Source: CAD feature listing. Evaluate the final solid. Frame: model axes, mm. Round coordinates to 2 decimals unless told otherwise and drop trailing zeros. Write each loop counter-clockwise with the first axis right and the second up, starting at its lowest first coordinate (ties: lowest second). Pieces come first, ordered by that corner, then holes. Notation, with made-up numbers: M 76.25,67 L 130.25,67 A8 cw 130.25,74 Z; hole C 86.5,72 d4. An arc over 180 degrees is marked long. Answer in a Markdown table with one row per item. Add a question column.
Item 1: Contact query for flat-ended pins moving along their axis: pin 1 (1.5 mm diameter, centred on y = 2.5, z = -1, fed in from +X); pin 2 (1 mm diameter, centred on y = 3, z = 1, fed in from -X); pin 3 (1 mm diameter, centred on y = 2.5, z = 0.5, fed in from -X). Output: stop coordinate, or through.
Item 2: Cut plane A-A on z = 0.7. Return loops of the section in (x, y).
Item 3: Mould query, pull axis Y, two halves, no side actions, for faces 1 (the face through (0, 0, 1.3)), 2 (the face through (0, 0, -1.3)). Classes: released by +Y, released by -Y, zero draft, split by the parting line, or undercut.
Item 4: Material intervals for probe 1 along Y at (x, z) = (-1.25, 1.1); probe 2 along Z at (x, y) = (-0.8, 0); probe 3 along Z at (x, y) = (-0.8, 1.5), sorted ascending.
from build123d import *

# Parameters (mm, degrees)
SKETCH1_W                = 3.6
SKETCH1_H                = 4.4
EXTRUDE1_DEPTH           = 1.3
EXTRUDE1_TAPER           = 7
EXTRUDE1_OTHER_WAY_DEPTH = 1.3
EXTRUDE1_OTHER_WAY_TAPER = 7
FILLET1_R                = 0.2
SKETCH3_W                = 0.4
SKETCH3_H                = 0.2
SKETCH7_R                = 0.3
EXTRUDE2_DEPTH           = 0.1
SKETCH5_W                = 0.4
SKETCH5_H                = 0.2


with BuildPart() as part:
    # Sketch1 → Extrude1 (new body)
    with BuildSketch(Plane.XY):
        Rectangle(SKETCH1_W, SKETCH1_H)
    extrude(amount=EXTRUDE1_DEPTH, taper=EXTRUDE1_TAPER)

    # Sketch1 → Extrude1 other way (add)
    with BuildSketch(Plane.XY):
        Rectangle(SKETCH1_W, SKETCH1_H)
    extrude(amount=-EXTRUDE1_OTHER_WAY_DEPTH, taper=EXTRUDE1_OTHER_WAY_TAPER)

    # Fillet1
    fillet1_edges = [part.edges().sort_by_distance(p)[0] for p in [
        (-1.640380071, 0, -1.3),
        (0, -2.040380071, -1.3),
        (1.640380071, 0, 1.3),
        (0, 2.040380071, 1.3),
        (-1.640380071, 0, 1.3),
        (0, -2.040380071, 1.3),
        (1.640380071, 0, -1.3),
        (0, 2.040380071, -1.3),
    ]]
    fillet(fillet1_edges, radius=FILLET1_R)

    # Sweep4: sweep along a path in Sketch4
    with BuildLine(Plane(origin=(0, 0, 0), x_dir=(0, 0, -1), z_dir=(1, 0, 0))) as sweep4_path:
        Line((0, 2.061944248), (0, 2.307301205))
        ThreePointArc((0, 2.307301205), (-0.04178036, 2.429639038), (-0.149665454, 2.500863685))
        Line((-0.149665454, 2.500863685), (-1.150334546, 2.761080563))
        ThreePointArc((-1.150334546, 2.761080563), (-1.25821964, 2.83230521), (-1.3, 2.954643043))
        Line((-1.3, 2.954643043), (-1.3, 3.5))
    # Sketch3 → Sweep4 (sweep)
    with BuildSketch(Plane(origin=(0, 2.061944248, 0), x_dir=(-1, 0, 0), z_dir=(0, 1, 0))):
        with Locations((1.27, 0)):
            Rectangle(SKETCH3_W, SKETCH3_H)
        with Locations((-1.27, 0)):
            Rectangle(SKETCH3_W, SKETCH3_H)
    sweep(path=sweep4_path.line)

    # Sketch7 → Extrude2 (cut)
    with BuildSketch(Plane(origin=(0, 0, -1.3), x_dir=(-1, 0, 0), z_dir=(0, 0, -1))):
        with Locations((1.02, 1.4)):
            Circle(SKETCH7_R)
    extrude(amount=-EXTRUDE2_DEPTH, mode=Mode.SUBTRACT)

    # Sweep3: sweep along a path in Sketch8
    with BuildLine(Plane(origin=(0, 0, 0), x_dir=(0, 0, -1), z_dir=(1, 0, 0))) as sweep3_path:
        Line((-1.3, -3.5), (-1.3, -2.954643043))
        ThreePointArc((-1.3, -2.954643043), (-1.25821964, -2.83230521), (-1.150334546, -2.761080563))
        Line((-1.150334546, -2.761080563), (-0.149665454, -2.500863685))
        ThreePointArc((-0.149665454, -2.500863685), (-0.04178036, -2.429639038), (0, -2.307301205))
        Line((0, -2.307301205), (0, -2.061944248))
    # Sketch5 → Sweep3 (sweep)
    with BuildSketch(Plane(origin=(0, -2.061944248, 0), x_dir=(-1, 0, 0), z_dir=(0, 1, 0))):
        with Locations((1.27, 0)):
            Rectangle(SKETCH5_W, SKETCH5_H)
        Rectangle(SKETCH5_W, SKETCH5_H)
        with Locations((-1.27, 0)):
            Rectangle(SKETCH5_W, SKETCH5_H)
    sweep(path=sweep3_path.line)


solid = part.part
Results below:
| question | item | result |
|---|---|---|
| 1 | pin 1 | x = 1.76 |
| 1 | pin 2 | x = -1.47 |
| 1 | pin 3 | x = -1.79 |
| 2 | outline | M -1.71,-2.11 L 1.71,-2.11 L 1.71,2.11 L -1.71,2.11 Z; M -1.47,-2.75 L -1.07,-2.75 L -1.07,-2.54 L -1.47,-2.54 Z; M -1.47,2.54 L -1.07,2.54 L -1.07,2.75 L -1.47,2.75 Z; M -0.2,-2.75 L 0.2,-2.75 L 0.2,-2.54 L -0.2,-2.54 Z; M 1.07,-2.75 L 1.47,-2.75 L 1.47,-2.54 L 1.07,-2.54 Z; M 1.07,2.54 L 1.47,2.54 L 1.47,2.75 L 1.07,2.75 Z |
| 3 | face 1 | undercut |
| 3 | face 2 | zero draft |
| 4 | probe 1 | -2.85 to -2.64, -2.06 to 2.06, 2.64 to 2.85 |
| 4 | probe 2 | -1.3 to 1.3 |
| 4 | probe 3 | -1.2 to 1.3 |
